Geometry check sheet. Reference: the model listing, model coordinates, mm. Give positions to 0.01 mm unless a question says otherwise; leave off trailing zeros. Loops run counter-clockwise (first coordinate to the right, second up) from the corner with the lowest first, then second, coordinate; pieces in that order, holes last. Notation, with made-up numbers: (17.5, -8.5) -> (28.5, -8.5) arc R9 ccw to (28.5, 3.5) -> close; hole circle Ø1 at (60.25, 71). An arc over 180 degrees is marked (long way). One line per question, with ' | ' between items.
from build123d import *

# Parameters (mm, degrees)
BOSS_EXTRUDE1_DEPTH = 20
SKETCH3_R           = 11
CUT_EXTRUDE1_DEPTH  = 42.979161497


with BuildPart() as part:
    # Sketch1 → Boss-Extrude1 (new body)
    with BuildSketch(Plane.XY):
        with BuildLine():
            Line((14.696938457, 3.5), (30, 3.5))
            Line((30, 3.5), (30, -3.5))
            Line((30, -3.5), (-30, -3.5))
            Line((-30, -3.5), (-30, 3.5))
            Line((-30, 3.5), (-14.696938457, 3.5))
            ThreePointArc((-14.696938457, 3.5), (0, 21.5), (14.696938457, 3.5))
        make_face()
    extrude(amount=BOSS_EXTRUDE1_DEPTH)

    # Sketch3 → Cut-Extrude1 (cut, through all)
    with BuildSketch(Plane.XY.offset(20)):
        with Locations((0.475039653, 7.440620043)):
            Circle(SKETCH3_R)
    extrude(amount=-CUT_EXTRUDE1_DEPTH, mode=Mode.SUBTRACT)


solid = part.part
Item 1: Release check for a two-part mould opening along Y. For faces 1 (the face through (0.94, 18.43, 10.14)), 2 (the face through (-30, 0, 10)), 3 (the face through (16, -3.5, 10)) record: pulls with the +Y half, pulls with the -Y half, needs draft (parallel to the pull), parting line crosses it, or undercut.
Result:
face 1: undercut | face 2: needs draft | face 3: pulls with the -Y half
Item 2: Scan lines: probe 1 along Y at (x, z) = (-18.5, 9); probe 2 along X at (y, z) = (8, 14); probe 3 along X at (y, z) = (17.5, 16.25). Record each from-to range of solid material in increasing order.
Result:
probe 1: -3.5 to 3.5 | probe 2: -14.92 to -10.51, 11.46 to 14.92 | probe 3: -10.2 to -3.98, 4.93 to 10.2
Item 3: Sectioned sample at C-C (x = -9). Record the cut outline in (y, z), plus the area to 3 significant figures.
Result:
outline: (-3.5, 0) -> (1.85, 0) -> (1.85, 20) -> (-3.5, 20) -> close; (13.03, 0) -> (18.5, 0) -> (18.5, 20) -> (13.03, 20) -> close | area: 216 mm2
Item 4: Sectioned sample at B-B (y = 7.5). Record the cut outline in (x, z), plus the area to 3 significant figures.
Result:
outline: (-14.97, 0) -> (-10.52, 0) -> (-10.52, 20) -> (-14.97, 20) -> close; (11.47, 0) -> (14.97, 0) -> (14.97, 20) -> (11.47, 20) -> close | area: 159 mm2
Item 5: Depth check by flat-ended pin: pin 1 Ø1 at (y, z) = (15, 10) entering from -X; pin 2 Ø4 at (x, z) = (-8.5, 10) entering from +Y; pin 3 Ø6 at (x, y) = (-19.5, 11) entering from -Z. Enter the tip coordinate at first touch or a pass-through.
Result:
pin 1: x = -12.69 | pin 2: y = 20.02 | pin 3: through
Item 6: Sectioned sample at A-A (z = 10.25). Record the cut outline in (x, y), plus the area to 3 significant figures.
Result:
outline: (-30, -3.5) -> (-0.67, -3.5) arc R11 cw (long way) to (1.62, -3.5) -> (30, -3.5) -> (30, 3.5) -> (14.7, 3.5) arc R15 ccw (long way) to (-14.7, 3.5) -> (-30, 3.5) -> close | area: 483 mm2
Item 7: Sectioned sample at D-D (x = -22). Record the cut outline in (y, z), plus the area to 3 significant figures.
Result:
outline: (-3.5, 0) -> (3.5, 0) -> (3.5, 20) -> (-3.5, 20) -> close | area: 140 mm2
